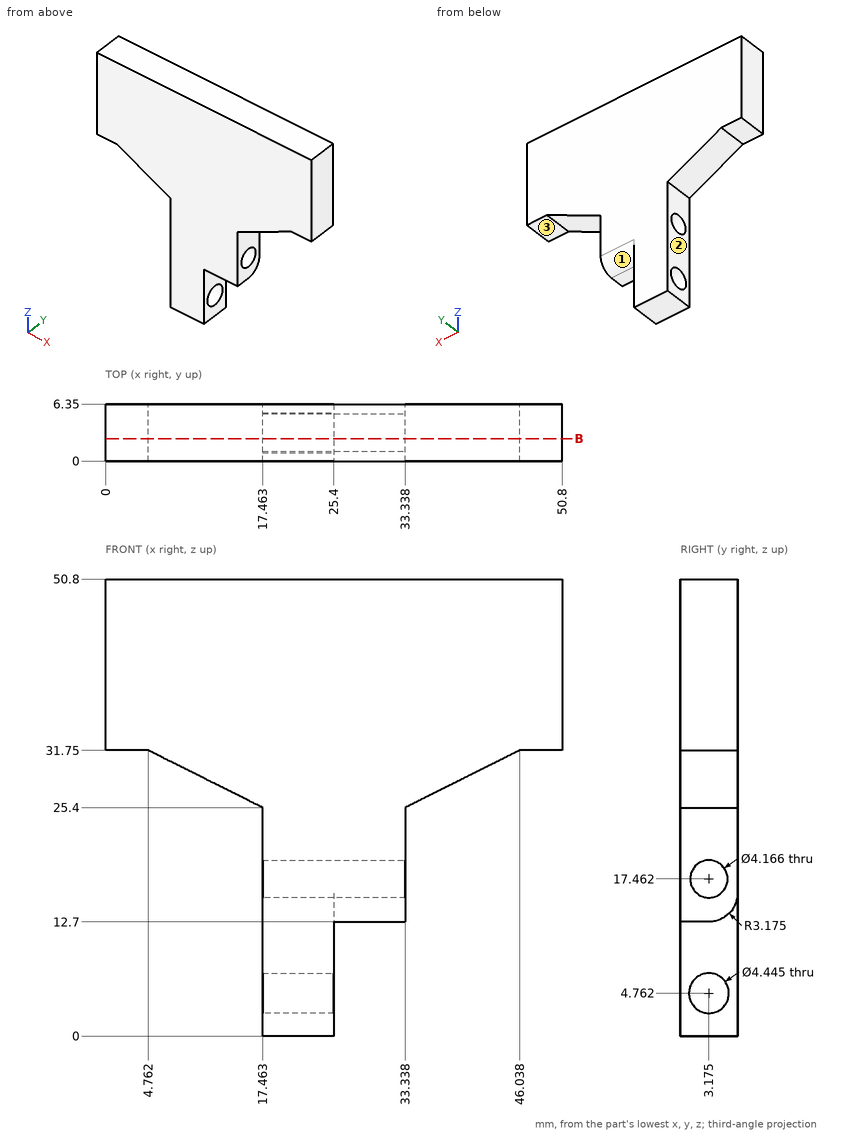
Part print with two shaded views. Sizes in mm from the minimum x, y, z corner. A direction names the side the tool comes from. Coordinates: 2 decimals unless noted, no trailing zeros. Write item = value, one per line. Start each with the question number.
1) 3-axis set-ups, long thin cutter, end or side, ignore diameter. For the marked faces 1, 2 and 3: which of +Z, -Z, +X, -X, +Y, -Y reach the whole face in a straight line?
2) Wall check: line 1 along Z through (x, y) = (24.5, 3.5) (1 decimal); line 2 along Z through (x, y) = (4, 1); line 3 along X through (y, z) = (3, 9). Give the ranges that are in metal, low to high. Write a range as from..to.
3) Saw through at B-B on y = 2.5. Count the separate pieces of the cut face and the enclosed holes in it, then the cut area to 3 significant figures.
4) Flat gauge pins, fed straight in: pin 1 Ø1.5 at (y, z) = (3, 26.5) entering from -X (1 decimal); pin 2 Ø2 at (y, z) = (1, 20) entering from +X; pin 3 Ø2.5 at (x, y) = (29, 1) entering from -Z; pin 4 Ø3.5 at (y, z) = (3.18, 4.76) entering from -X. Where does each tip first touch, or does it go through?
From the geometry:
q1.face_1 = -Z, +X, +Y
q1.face_2 = -Z, -X, +Y, -Y
q1.face_3 = -Z, +X, +Y, -Y
q2.line_1 = 0..2.6, 7..15.4, 19.5..50.8
q2.line_2 = 31.75..50.8
q2.line_3 = 17.46..25.4
q3.separate_pieces = 3
q3.enclosed_holes = 0
q3.area = 1,360 mm^2
q4.pin_1 = 13.8
q4.pin_2 = 33.34
q4.pin_3 = 12.7
q4.pin_4 = through
